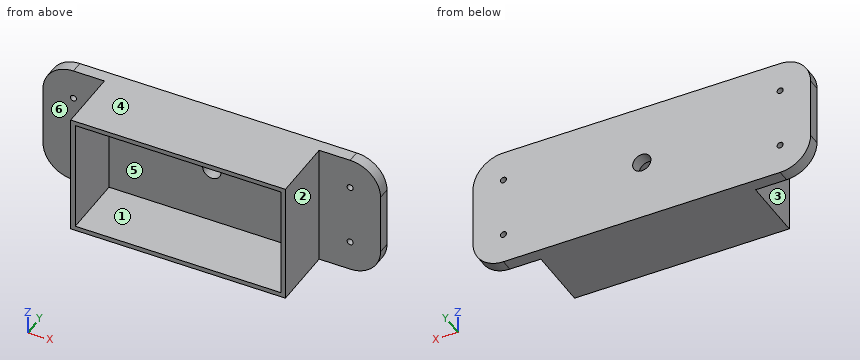
from build123d import *

# Parameters (mm, degrees)
SKETCH1_R           = 1
BOSS_EXTRUDE1_DEPTH = 4
BOSS_EXTRUDE3_DEPTH = 25
SKETCH3_R           = 3
CUT_EXTRUDE1_DEPTH  = 20


with BuildPart() as part:
    # Sketch1 → Boss-Extrude1 (new body)
    with BuildSketch(Plane(origin=(0, 0, 0), x_dir=(1, 0, 0), z_dir=(0, 1, 0))):
        with BuildLine():
            Line((-35.5, 20), (-35.5, 0))
            Line((-35.5, 0), (-35.5, -20))
            Line((-35.5, -20), (45.5, -20))
            ThreePointArc((45.5, -20), (52.571067812, -17.071067812), (55.5, -10))
            Line((55.5, -10), (55.5, 10))
            ThreePointArc((55.5, 10), (52.571067812, 17.071067812), (45.5, 20))
            Line((45.5, 20), (-35.5, 20))
        make_face()
        with Locations((45.5, -10)):
            Circle(SKETCH1_R, mode=Mode.SUBTRACT)
        Circle(SKETCH1_R, mode=Mode.SUBTRACT)
        with Locations((45.5, 10)):
            Circle(SKETCH1_R, mode=Mode.SUBTRACT)
        with BuildLine():
            Line((-35.5, -20), (-35.5, 0))
            Line((-35.5, 0), (-35.5, 20))
            Line((-35.5, 20), (-45.5, 20))
            ThreePointArc((-45.5, 20), (-52.571067812, 17.071067812), (-55.5, 10))
            Line((-55.5, 10), (-55.5, 0))
            Line((-55.5, 0), (-55.5, -10))
            ThreePointArc((-55.5, -10), (-52.571067812, -17.071067812), (-45.5, -20))
            Line((-45.5, -20), (-35.5, -20))
        make_face()
        with Locations((-45.5, -10)):
            Circle(SKETCH1_R, mode=Mode.SUBTRACT)
        with Locations((-45.5, 10)):
            Circle(SKETCH1_R, mode=Mode.SUBTRACT)
    extrude(amount=BOSS_EXTRUDE1_DEPTH)

    # Sketch2 → Boss-Extrude3 (add)
    with BuildSketch(Plane(origin=(0, 4, 0), x_dir=(1, 0, 0), z_dir=(0, 1, 0))):
        Polygon((-35.3, 0), (-35.3, -20), (35.3, -20), (35.3, 0), (35.3, 20), (-35.3, 20), align=None)
        Polygon((33.8, -18.5), (-33.8, -18.5), (-33.8, 0), (-33.8, 18.5), (33.8, 18.5), (33.8, 0), align=None, mode=Mode.SUBTRACT)
    extrude(amount=-BOSS_EXTRUDE3_DEPTH)

    # Sketch3 → Cut-Extrude1 (cut)
    with BuildSketch(Plane(origin=(0, 4, 0), x_dir=(1, 0, 0), z_dir=(0, 1, 0))):
        Circle(SKETCH3_R)
    extrude(amount=-CUT_EXTRUDE1_DEPTH, mode=Mode.SUBTRACT)


solid = part.part
Geometry: final body of the model. Coordinates: model frame, mm. Face numbers are marked on the shaded views. A direction names the side the tool comes from. Give positions to 0.01 mm unless a question says otherwise; leave off trailing zeros. Order: outer loops, then holes, each group sorted by start corner. A loop starts at its lowest first (then second) coordinate and runs counter-clockwise, first axis right, second up. Notation, with made-up numbers: (-27.75, 26) -> (22.25, 26) arc R19 cw to (22.25, 60) -> close; hole circle Ø2 at (3, 78). An arc over 180 degrees is marked (long way). Write each question's results on one line, items separated by ' | '.
1) Line query: line 1 along X through (y, z) = (1.75, 10); line 2 along Z through (x, y) = (45.5, 1.35); line 3 along X through (y, z) = (-6.5, -15). Output: solid intervals per line, ascending.
Geometry says:
line 1: x = -55.5 to -46.5, -44.5 to 44.5, 46.5 to 55.5 | line 2: z = -20 to -11, -9 to 9, 11 to 20 | line 3: x = -35.3 to -33.8, 33.8 to 35.3
2) Cut plane C-C (y = -14). Output: boundary loops of the cut face in (x, z).
Geometry says:
outline: (-35.3, -20) -> (35.3, -20) -> (35.3, 20) -> (-35.3, 20) -> close; hole (-33.8, -18.5) -> (33.8, -18.5) -> (33.8, 18.5) -> (-33.8, 18.5) -> close
3) Cut plane A-A (z = 0). Output: boundary loops of the cut face in (x, y).
Geometry says:
outline: (-55.5, 0) -> (-35.3, 0) -> (-35.3, -21) -> (-33.8, -21) -> (-33.8, 0) -> (-3, 0) -> (-3, 4) -> (-55.5, 4) -> close; (3, 0) -> (33.8, 0) -> (33.8, -21) -> (35.3, -21) -> (35.3, 0) -> (55.5, 0) -> (55.5, 4) -> (3, 4) -> close
4) Cut plane D-D (x = -24). Output: boundary loops of the cut face in (y, z).
Geometry says:
outline: (-21, -20) -> (4, -20) -> (4, 20) -> (-21, 20) -> (-21, 18.5) -> (0, 18.5) -> (0, -18.5) -> (-21, -18.5) -> close
5) Set-up query: the marked faces 1, 2 and 3. Return all of +Z, -Z, +X, -X, +Y, -Y with unobstructed straight access to the full face (end or side cutting, diameter ignored); none if empty.
Geometry says:
face 1: -Y | face 2: +Z, -Z, +X, -Y | face 3: +Z, -Z, -X, -Y
6) First-contact query: pin 1 Ø16 at (x, z) = (-49, -5) entering from -Y; pin 2 Ø6.5 at (y, z) = (-11.5, 9) entering from -X; pin 3 Ø10.5 at (y, z) = (-14.5, -1.5) entering from +X. Flat tips, straight axial feed; report the tip coordinate or a pass-through.
Geometry says:
pin 1: stops at y = 0 | pin 2: stops at x = -35.3 | pin 3: stops at x = 35.3
7) Draft query along Z for the marked faces 4, 5 and 6. Return one class per face: released by +Z, released by -Z, zero draft, split by the parting line, or undercut.
Geometry says:
face 4: released by +Z | face 5: undercut | face 6: zero draft
8) Cut plane B-B (x = 0). Output: boundary loops of the cut face in (y, z).
Geometry says:
outline: (-21, -20) -> (4, -20) -> (4, -3) -> (0, -3) -> (0, -18.5) -> (-21, -18.5) -> close; (-21, 18.5) -> (0, 18.5) -> (0, 3) -> (4, 3) -> (4, 20) -> (-21, 20) -> close
